The model under review builds one solid part; all positions refer to its coordinate system, in mm. A direction names the side the tool comes from. Round coordinates to 2 decimals unless told otherwise and drop trailing zeros. Order: outer loops, then holes, each group sorted by start corner. A loop starts at its lowest first (then second) coordinate and runs counter-clockwise, first axis right, second up. Notation, with made-up numbers: M -12,59.25 L -5,59.25 A17 ccw -5,85.25 Z; hole C 6,89.25 d8. An arc over 180 degrees is marked long. Answer as a JSON object with one key per item and string values. Group by question number.
1) For faces 1 (the flat face through (0, 13.5, 2)), 2 (the flat face through (0, -10.5, 3)), 3 (the flat face through (-12, 0, 4)), list the 3-axis set-ups (+Z, -Z, +X, -X, +Y, -Y) from which the entire face can be reached by the end or side of a thin tool; tool diameter is ignored.
2) To check wall thickness, follow line 1 (Y direction, x = -8, z = 1.95); line 2 (Y direction, x = 4.25, z = 4.45); line 3 (Y direction, x = -8, z = 1). State the ranges of each line that lie inside material, in increasing order.
3) Consider section A-A, the plane z = 0.6. Write out the cut boundary in (x, y).
4) Consider section D-D, the plane x = -2.25. Write out the cut boundary in (y, z), then the cut area to 3 significant figures.
5) The part is to be moulded in two halves that separate along Y. For faces 4 (the cylindrical face through (12.4, 12.93, 2.54)), 5 (the flat face through (0, -12, 5)), 6 (the flat face through (0, 0, 1.5)), say which applies: +Y half, -Y half, draft (parallel to the pull), parting line (faces both ways), or undercut.
6) Insertion check: pin 1 Ø6 at (x, y) = (7, 5.5) entering from -Z; pin 2 Ø3 at (x, z) = (-4, 3) entering from -Y; pin 3 Ø1.2 at (x, y) = (-12, 0.5) entering from +Z; pin 4 Ø1.5 at (x, z) = (9.5, 4) entering from -Y. Each pin has a flat end and moves straight along its axis. Give the tip position at first contact, or say it passes through.
7) Consider section C-C, the plane y = -7. Write out the cut boundary in (x, z), then the cut area to 3 significant figures.
8) Consider section B-B, the plane x = -8. Write out the cut boundary in (y, z), then the cut area to 3 significant figures.
```python
from build123d import *

# Parameters (mm, degrees)
ESQUISSE1_R             = 1
ESQUISSE1_W             = 21
ESQUISSE1_H             = 21
BOSS_EXTRU_1_DEPTH      = 5
ESQUISSE2_W             = 21
ESQUISSE2_H             = 21
BOSS_EXTRU_2_DEPTH      = 1.5
ESQUISSE3_W             = 2.5
ESQUISSE3_H             = 19
ENL_V_MAT_EXTRU_1_DEPTH = 1
CONG_1_R                = 2
CONG_2_R                = 2
CONG_3_R                = 0.5


with BuildPart() as part:
    # Esquisse1 → Boss.-Extru.1 (new body)
    with BuildSketch(Plane.XY):
        with BuildLine():
            Line((13, 13.5), (9.732050808, 13.5))
            ThreePointArc((9.732050808, 13.5), (8, 14.5), (6.267949192, 13.5))
            Line((6.267949192, 13.5), (-6.267949192, 13.5))
            ThreePointArc((-6.267949192, 13.5), (-8, 14.5), (-9.732050808, 13.5))
            Line((-9.732050808, 13.5), (-13, 13.5))
            Line((-13, 13.5), (-13, -13.5))
            Line((-13, -13.5), (-9.732050808, -13.5))
            ThreePointArc((-9.732050808, -13.5), (-8, -14.5), (-6.267949192, -13.5))
            Line((-6.267949192, -13.5), (6.267949192, -13.5))
            ThreePointArc((6.267949192, -13.5), (8, -14.5), (9.732050808, -13.5))
            Line((9.732050808, -13.5), (13, -13.5))
            Line((13, -13.5), (13, 13.5))
        make_face()
        with Locations((-8, 12.5)):
            Circle(ESQUISSE1_R, mode=Mode.SUBTRACT)
        with Locations(Location((8, 12.5, 0), (0, 0, 180))):
            Circle(ESQUISSE1_R, mode=Mode.SUBTRACT)
        with Locations((8, -12.5)):
            Circle(ESQUISSE1_R, mode=Mode.SUBTRACT)
        with Locations(Location((-8, -12.5, 0), (0, 0, 180))):
            Circle(ESQUISSE1_R, mode=Mode.SUBTRACT)
        Rectangle(ESQUISSE1_W, ESQUISSE1_H, mode=Mode.SUBTRACT)
    extrude(amount=BOSS_EXTRU_1_DEPTH)

    # Esquisse2 → Boss.-Extru.2 (add)
    with BuildSketch(Plane(origin=(0, 0, 0), x_dir=(-1, 0, 0), z_dir=(0, 0, -1))):
        Rectangle(ESQUISSE2_W, ESQUISSE2_H)
    extrude(amount=-BOSS_EXTRU_2_DEPTH)

    # Esquisse3 → Enlèv. mat.-Extru.1 (cut)
    with BuildSketch(Plane.XY.offset(5)):
        with Locations((-11.75, 0)):
            Rectangle(ESQUISSE3_W, ESQUISSE3_H)
        with Locations((11.75, 0)):
            Rectangle(ESQUISSE3_W, ESQUISSE3_H)
    extrude(amount=-ENL_V_MAT_EXTRU_1_DEPTH, mode=Mode.SUBTRACT)

    # Congé1
    cong_1_edges = [part.edges().sort_by_distance(p)[0] for p in [
        (-13, -13.5, 2.5),
        (-13, 13.5, 2.5),
        (13, 13.5, 2.5),
        (13, -13.5, 2.5),
    ]]
    fillet(cong_1_edges, radius=CONG_1_R)

    # Congé2
    cong_2_edges = [part.edges().sort_by_distance(p)[0] for p in [
        (-9.732050808, 13.5, 2.5),
        (-6.267949192, 13.5, 2.5),
        (6.267949192, 13.5, 2.5),
        (9.732050808, 13.5, 2.5),
        (9.732050808, -13.5, 2.5),
        (6.267949192, -13.5, 2.5),
        (-6.267949192, -13.5, 2.5),
        (-9.732050808, -13.5, 2.5),
    ]]
    fillet(cong_2_edges, radius=CONG_2_R)

    # Congé3
    cong_3_edges = [part.edges().sort_by_distance(p)[0] for p in [
        (13, -9.5, 4.5),
        (-13, 9.5, 4.5),
        (-13, -9.5, 4.5),
        (-10.5, -9.5, 4.5),
        (-10.5, 9.5, 4.5),
        (10.5, 9.5, 4.5),
        (10.5, -9.5, 4.5),
        (13, 0, 4),
        (-13, 0, 4),
        (-10.5, 0, 4),
        (10.5, 0, 4),
        (13, 9.5, 4.5),
        (11.75, -9.5, 4),
        (11.75, 9.5, 4),
        (-11.75, 9.5, 4),
        (-11.75, -9.5, 4),
        (-10.5, -10.5, 3.25),
        (10.5, -10.5, 3.25),
        (10.5, 10.5, 3.25),
        (-10.5, 10.5, 3.25),
    ]]
    fillet(cong_3_edges, radius=CONG_3_R - 0.0001)  # a hair under: the kernel refuses the full size


solid = part.part
```
Results list:
{
 "1": {"face 1": "+Z, -Z, +Y", "face 2": "+Z", "face 3": "+Z, +X, -X"},
 "2": {"line 1": "-14.5 to -13.5, -11.5 to -10.5, 10.5 to 11.5, 13.5 to 14.5", "line 2": "-13.5 to -10.5, 10.5 to 13.5", "line 3": "-14.5 to -13.5, -11.5 to 11.5, 13.5 to 14.5"},
 "3": {"outline": "M -13,-11.5 A2 ccw -11,-13.5 L -10.65,-13.5 A2 cw -9.32,-14 A2 ccw -6.68,-14 A2 cw -5.35,-13.5 L 5.35,-13.5 A2 cw 6.68,-14 A2 ccw 9.32,-14 A2 cw 10.65,-13.5 L 11,-13.5 A2 ccw 13,-11.5 L 13,11.5 A2 ccw 11,13.5 L 10.65,13.5 A2 cw 9.32,14 A2 ccw 6.68,14 A2 cw 5.35,13.5 L -5.35,13.5 A2 cw -6.68,14 A2 ccw -9.32,14 A2 cw -10.65,13.5 L -11,13.5 A2 ccw -13,11.5 Z; hole C -8,-12.5 d2; hole C -8,12.5 d2; hole C 8,-12.5 d2; hole C 8,12.5 d2"},
 "4": {"outline": "M -13.5,0 L 13.5,0 L 13.5,5 L 10.5,5 L 10.5,1.5 L -10.5,1.5 L -10.5,5 L -13.5,5 Z", "area": "61.5 mm^2"},
 "5": {"face 4": "+Y half", "face 5": "draft", "face 6": "undercut"},
 "6": {"pin 1": "z = 0", "pin 2": "y = -13.51", "pin 3": "z = 4", "pin 4": "y = -14.35"},
 "7": {"outline": "M -13,0 L 13,0 L 13,3.5 A0.5 ccw 12.5,4 L 11,4 A0.5 ccw 10.5,3.5 L 10.5,1.5 L -10.5,1.5 L -10.5,3.5 A0.5 ccw -11,4 L -12.5,4 A0.5 ccw -13,3.5 Z", "area": "51.3 mm^2"},
 "8": {"outline": "M -14.5,0 L -13.5,0 L -13.5,5 L -14.5,5 Z; M -11.5,0 L 11.5,0 L 11.5,5 L 10.5,5 L 10.5,1.5 L -10.5,1.5 L -10.5,5 L -11.5,5 Z; M 13.5,0 L 14.5,0 L 14.5,5 L 13.5,5 Z", "area": "51.5 mm^2"}
}
